Here's how the part is built. I have some questions about the finished solid (model axes, mm). A direction names the side the tool comes from. Coordinates: 2 decimals unless noted, no trailing zeros. Write each loop counter-clockwise with the first axis right and the second up, starting at its lowest first coordinate (ties: lowest second). Pieces come first, ordered by that corner, then holes.
Item 1: Please list where these lines run through material, in increasing order: line 1 (Y direction, x = -2.5, z = 0.25); line 2 (Z direction, x = 1, y = 6); line 3 (X direction, y = -6, z = 5.5).
Item 2: I'm going to push flat-ended pins straight in: P1, Ø8, axis at x = -13.5, y = -10, coming from the -Z side; P2, Ø3, axis at y = -9, z = 0, coming from the -X side; P3, Ø4, axis at x = -6.5, z = -7.5, coming from the +Y side; P4, Ø6, axis at x = -18.5, z = 3, coming from the -Y side. Where does each tip first touch, or does it pass through?
Item 3: If we mould it in two halves opening along X, with no side actions, what happens to faces 4 (the face through (25, -6, 0)), 5 (the face through (-30, 0, 0)), 6 (the face through (-25, -14, 0))? For each: pulls with the +X half, pulls with the -X half, needs draft (parallel to the pull), parting line crosses it, or undercut.
Item 4: I want a section at A-A (y = 0). Please give me the cut outline in (x, z).
Item 5: I want a section at D-D (x = -25). Please give me the cut outline in (y, z), and give its area (3 significant figures).
Item 6: For faces 1 (the face through (-27, -12, 0)), 2 (the face through (25.35, 2, -6)), 3 (the face through (26.95, -1.73, 7.81)), which set-ups out of +Z, -Z, +X, -X, +Y, -Y let a thin tool reach every point of the face, with its end or its side?
Item 7: I want a section at C-C (x = 15). Please give me the cut outline in (y, z), and give its area (3 significant figures).
Item 8: I want a section at B-B (z = 0). Please give me the cut outline in (x, y).
from build123d import *

# Parameters (mm, degrees)
SKETCH1_W           = 54
SKETCH1_H           = 10
SKETCH3_R           = 2
BOSS_EXTRUDE1_DEPTH = 14
SKETCH4_W           = 6
SKETCH4_H           = 8
SKETCH5_W           = 1.35
SKETCH5_H           = 2


with BuildPart() as part:
    # Sketch1 → Revolve1 (revolve)
    with BuildSketch(Plane.XY):
        with Locations((-3, 5)):
            Rectangle(SKETCH1_W, SKETCH1_H)
    revolve(axis=Axis((24, 0, 0), (-1, 0, 0)))

    # Sketch2 → Cut-Revolve1 (revolve, cut)
    with BuildSketch(Plane.XY):
        Polygon((-30, 8.5), (-28.5, 10), (-30, 10), align=None)
    revolve(axis=Axis((49, 0, 0), (-1, 0, 0)), mode=Mode.SUBTRACT)

    # Sketch3 → Boss-Extrude1 (add)
    with BuildSketch(Plane(origin=(0, 0, 0), x_dir=(1, 0, 0), z_dir=(0, 1, 0))):
        with Locations((-25, 0)):
            Circle(SKETCH3_R)
    extrude(amount=-BOSS_EXTRUDE1_DEPTH)

    # Sketch4 → Revolve2 (revolve)
    with BuildSketch(Plane.XY):
        with Locations((27, 4)):
            Rectangle(SKETCH4_W, SKETCH4_H)
    revolve(axis=Axis((30, 0, 0), (-1, 0, 0)))

    # Sketch5 → Cut-Revolve2 (revolve, cut)
    with BuildSketch(Plane.XY):
        with Locations((24.675, 7)):
            Rectangle(SKETCH5_W, SKETCH5_H)
    revolve(axis=Axis((49, 0, 0), (-1, 0, 0)), mode=Mode.SUBTRACT)

    # Sketch6 → Cut-Revolve3 (revolve, cut)
    with BuildSketch(Plane.XY):
        Polygon((28.5, 8), (30, 6.5), (30, 8), align=None)
    revolve(axis=Axis((49, 0, 0), (-1, 0, 0)), mode=Mode.SUBTRACT)


solid = part.part
Answer:
1. line 1: y = -10 to 10
1. line 2: z = -8 to 8
1. line 3: x = -30 to 24
2. P1: stops at z = -8
2. P2: stops at x = -30
2. P3: stops at y = 8.35
2. P4: stops at y = -10
3. face 4: undercut
3. face 5: pulls with the -X half
3. face 6: needs draft
4. outline: (-30, -8.5) - (-28.5, -10) - (24, -10) - (24, -6) - (25.35, -6) - (25.35, -8) - (28.5, -8) - (30, -6.5) - (30, 6.5) - (28.5, 8) - (25.35, 8) - (25.35, 6) - (24, 6) - (24, 10) - (-28.5, 10) - (-30, 8.5) - close
5. outline: (-14, -2) - (-9.8, -2) arc R10 ccw (long way) to (-9.8, 2) - (-14, 2) - close
5. area: 330 mm2
6. face 1: -Y
6. face 2: none
6. face 3: +X
7. outline: circle Ø20 at (0, 0)
7. area: 314 mm2
8. outline: (-30, -8.5) - (-28.5, -10) - (-27, -10) - (-27, -14) - (-23, -14) - (-23, -10) - (24, -10) - (24, -6) - (25.35, -6) - (25.35, -8) - (28.5, -8) - (30, -6.5) - (30, 6.5) - (28.5, 8) - (25.35, 8) - (25.35, 6) - (24, 6) - (24, 10) - (-28.5, 10) - (-30, 8.5) - close
